Geometry check sheet. Reference: the model listing, model coordinates, mm. Face numbers are marked on the shaded views. A direction names the side the tool comes from. Round coordinates to 2 decimals unless told otherwise and drop trailing zeros. Loops run counter-clockwise (first coordinate to the right, second up) from the corner with the lowest first, then second, coordinate; pieces in that order, holes last. Notation, with made-up numbers: (-1, 20) - (15, 20) arc R8 cw to (15, 28) - close; hole circle Ø2 at (9, 77.5). An arc over 180 degrees is marked (long way). Answer in a Markdown table with one row per item. Add a question column.
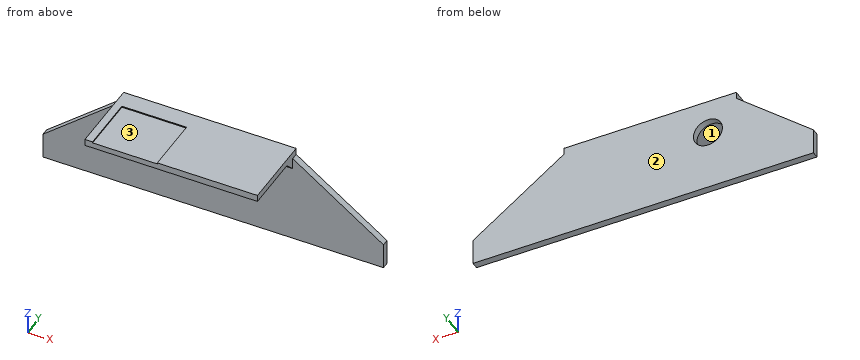
```python
from build123d import *

# Parameters (mm, degrees)
F1_DEPTH  = 6
F2_W      = 152
F2_H      = 6
F3_DEPTH  = 60
F4_W      = 57
F4_H      = 50
F5_DEPTH  = 1
F6_W      = 152
F6_H      = 10
F7_DEPTH  = 10
F9_DEPTH  = 160
F10_R     = 12.75
F11_DEPTH = 25


with BuildPart() as f1:
    # F0 (on Front) → F1 (new body)
    with BuildSketch(Plane.XZ):
        Polygon((-65.014175, 23), (-65.014175, 0), (234.985825, 0), (234.985825, 23), (154.985825, 80), (154.985825, 86), (2.985825, 86), (2.985825, 80), align=None)
    extrude(amount=F1_DEPTH)

    # F2 (on face) → F3 (join)
    with BuildSketch(Plane.XZ.offset(6)):
        with Locations((78.985825, 83)):
            Rectangle(F2_W, F2_H)
    extrude(amount=F3_DEPTH)

    # F4 (on face) → F5 (cut)
    with BuildSketch(Plane.XY.offset(86)):
        with Locations((38.185825, -41)):
            Rectangle(F4_W, F4_H)
    extrude(amount=-F5_DEPTH, mode=Mode.SUBTRACT)

    # F6 (on face) → F7 (join)
    with BuildSketch(Plane(origin=(0, 0, 80), x_dir=(1, 0, 0), z_dir=(0, 0, -1))):
        with Locations((78.985825, 11)):
            Rectangle(F6_W, F6_H)
    extrude(amount=F7_DEPTH)

    # F8 (on face) → F9 (cut)
    with BuildSketch(Plane(origin=(2.985825, 0, 0), x_dir=(0, -1, 0), z_dir=(-1, 0, 0))):
        Polygon((16, 70), (16, 80), (6, 70), align=None)
    extrude(amount=-F9_DEPTH, mode=Mode.SUBTRACT)

    # F10 (on face) → F11 (cut)
    with BuildSketch(Plane.XZ.offset(6)):
        with Locations((27.985825, 55)):
            Circle(F10_R)
    extrude(amount=-F11_DEPTH, mode=Mode.SUBTRACT)


solid = f1.part
```
Q1. Scan lines: line 1 (Y direction, x = 171.5, z = 24.5); line 2 (X direction, y = -4, z = 65); line 3 (Z direction, x = 45, y = -58.5). Record each from-to range of solid material in increasing order. Write a range as from..to.
Q2. Cross-section at A-A, the plane z = 63. Enter the section's corners in (x, y).
Q3. Cross-section at D-D, the plane z = 10.5. Enter the section's corners in (x, y), plus the area to 3 significant figures.
Q4. Depth check by flat-ended pin: P1, Ø15, axis at x = 29.5, y = -48, coming from the +Z side; P2, Ø17.5, axis at y = -42, z = 81, coming from the +X side; P3, Ø0.8, axis at y = -42, z = 85.5, coming from the -X side. Enter the tip coordinate at first touch or a pass-through.
Q5. Cross-section at C-C, the plane x = 132. Enter the section's corners in (y, z), plus the area to 3 significant figures.
Q6. Set-up check for the marked faces 1, 2 and 3: record each of +Z, -Z, +X, -X, +Y, -Y from which the full face is reachable in a straight line by a thin tool's end or side.
Q7. Cross-section at B-B, the plane y = -53.5. Enter the section's corners in (x, z).
Check sheet entries:
| question | item | result |
|---|---|---|
| 1 | line 1 | -6..0 |
| 1 | line 2 | -14.91..20.08, 35.9..176.04 |
| 1 | line 3 | 80..85 |
| 2 | outline | (-17.29, -6) - (18.06, -6) - (18.06, 0) - (-17.29, 0) - close; (37.91, -6) - (178.85, -6) - (178.85, 0) - (37.91, 0) - close |
| 3 | outline | (-65.01, -6) - (234.99, -6) - (234.99, 0) - (-65.01, 0) - close |
| 3 | area | 1,800 mm² |
| 4 | P1 | z = 85 |
| 4 | P2 | x = 154.99 |
| 4 | P3 | x = 2.99 |
| 5 | outline | (-66, 80) - (-16, 80) - (-6, 70) - (-6, 0) - (0, 0) - (0, 86) - (-66, 86) - close |
| 5 | area | 926 mm² |
| 6 | face 1 | -Z, +X, -X, -Y |
| 6 | face 2 | +Z, -Z, +X, -X, +Y |
| 6 | face 3 | +Z, -Y |
| 7 | outline | (2.99, 80) - (154.99, 80) - (154.99, 86) - (66.69, 86) - (66.69, 85) - (9.69, 85) - (9.69, 86) - (2.99, 86) - close |
